Source: CAD feature listing. Evaluate the final solid. Frame: model axes, mm. Face numbers are marked on the shaded views. A direction names the side the tool comes from. Give positions to 0.01 mm unless a question says otherwise; leave off trailing zeros. Order: outer loops, then holes, each group sorted by start corner. A loop starts at its lowest first (then second) coordinate and runs counter-clockwise, first axis right, second up. Notation, with made-up numbers: M -27.75,72 L 21.25,72 A15 ccw 21.25,90 Z; hole C -24,79 d10. An arc over 180 degrees is marked long. Return JSON: item names as keys, results as strings.
from build123d import *

# Parameters (mm, degrees)
F0_W          = 210
F0_H          = 225
F1_DEPTH      = 25
F3_DEPTH      = 95
F4_R          = 37.5
F5_DEPTH      = 10
F5_DEPTH_BACK = 127
F6_R          = 40
F7_DEPTH      = 10
F7_DEPTH_BACK = 127
F8_W          = 60
F8_H          = 60
F9_DEPTH      = 10


with BuildPart() as f1:
    # F0 (on Top) → F1 (new body)
    with BuildSketch(Plane.XY):
        Rectangle(F0_W, F0_H)
    extrude(amount=F1_DEPTH)

    # F2 (on face) → F3 (join)
    with BuildSketch(Plane.XY.offset(25)):
        with BuildLine():
            Line((-71, -32.5), (-71, -112.5))
            Line((-71, -112.5), (-56, -112.5))
            Line((-56, -112.5), (-56, -46.481817))
            ThreePointArc((-56, -46.481817), (7.488853, -14.988853), (38.981817, 48.5))
            Line((38.981817, 48.5), (105, 48.5))
            Line((105, 48.5), (105, 63.5))
            Line((105, 63.5), (25, 63.5))
            ThreePointArc((25, 63.5), (-3.117749, -4.382251), (-71, -32.5))
        make_face()
    extrude(amount=F3_DEPTH)

    # F4 (on face) → F5 (join, two sides)
    with BuildSketch(Plane.XZ.offset(112.5)) as f5_sk:
        with Locations((-63.5, 120)):
            Circle(F4_R)
    extrude(amount=F5_DEPTH)
    extrude(f5_sk.sketch, amount=-F5_DEPTH_BACK)

    # F6 (on face) → F7 (join, two sides)
    with BuildSketch(Plane.YZ.offset(105)) as f7_sk:
        with Locations((56, 120)):
            Circle(F6_R)
    extrude(amount=F7_DEPTH)
    extrude(f7_sk.sketch, amount=-F7_DEPTH_BACK)

    # F8 (on face) → F9 (join)
    with BuildSketch(Plane.XY.offset(25)):
        with Locations((75, -82.5)):
            Rectangle(F8_W, F8_H)
    extrude(amount=F9_DEPTH)


solid = f1.part
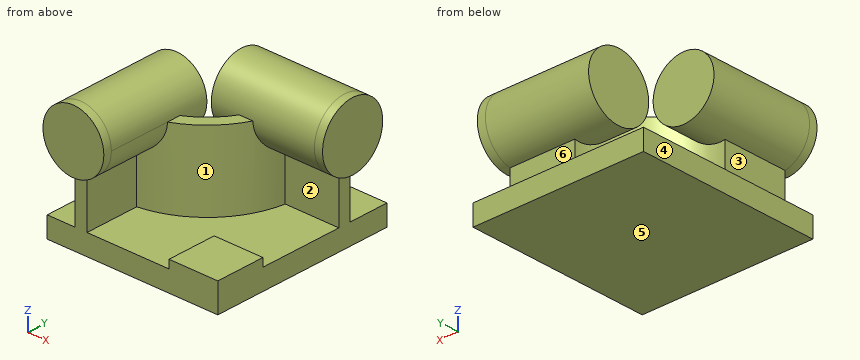
1. Section query B-B (y = 79.5). Return loops of the section in (x, z).
Evaluation:
{"outline": "M -105,0 L 105,0 L 105,25 L -105,25 Z; M -22,87.63 L 115,87.63 L 115,152.37 L -22,152.37 Z"}
2. Section query D-D (z = 106.5). Return loops of the section in (x, y).
Evaluation:
{"outline": "M -98.49,-122.5 L -28.51,-122.5 L -28.51,-39.05 A111 ccw 30.4,18.35 L 115,18.35 L 115,93.65 L -22,93.65 L -22,18.35 L 13.72,18.35 A96 cw -28.51,-22.59 L -28.51,14.5 L -98.49,14.5 Z"}
3. Section query C-C (y = -72). Return loops of the section in (x, z).
Evaluation:
{"outline": "M -105,0 L 105,0 L 105,35 L 45,35 L 45,25 L -56,25 L -56,83.26 A37.5 ccw long -71,83.26 L -71,25 L -105,25 Z"}
4. Set-up query: the marked faces 1, 2 and 3. Return all of +Z, -Z, +X, -X, +Y, -Y with unobstructed straight access to the full face (end or side cutting, diameter ignored); none if empty.
Evaluation:
{"face 1": "+X, -Y", "face 2": "+X", "face 3": "-X, +Y, -Y"}
5. First-contact query: pin 1 (16.5 mm diameter, centred on x = 74.5, z = 54.5, fed in from +Y); pin 2 (1 mm diameter, centred on y = -57, z = 44, fed in from -X); pin 3 (4 mm diameter, centred on y = -68.5, z = 34.5, fed in from +X); pin 4 (6 mm diameter, centred on x = 18.5, y = 43.5, fed in from -Z). Flat tips, straight axial feed; report the tip coordinate or a pass-through.
Evaluation:
{"pin 1": "stops at y = 63.5", "pin 2": "stops at x = -71", "pin 3": "stops at x = 105", "pin 4": "stops at z = 0"}
6. Section query A-A (x = 70). Return loops of the section in (y, z).
Evaluation:
{"outline": "M -112.5,0 L 112.5,0 L 112.5,25 L 63.5,25 L 63.5,80.71 A40 ccw long 48.5,80.71 L 48.5,25 L -52.5,25 L -52.5,35 L -112.5,35 Z"}
7. Draft query along Z for the marked faces 4, 5 and 6. Return one class per face: pulls with the +Z half, pulls with the -Z half, needs draft (parallel to the pull), parting line crosses it, or undercut.
Evaluation:
{"face 4": "needs draft", "face 5": "pulls with the -Z half", "face 6": "undercut"}
8. Ray query, probe 1 along X at (y, z) = (-74, 46.5); probe 2 along X at (y, z) = (33, 139.5); probe 3 along Y at (x, z) = (8, 93). Return the intervals inside material, ascending.
Evaluation:
{"probe 1": "x = -71 to -56", "probe 2": "x = -22 to 115", "probe 3": "y = -14.47 to 8.96, 26.49 to 85.51"}
